from build123d import *

# Parameters (mm, degrees)
F1_DEPTH = 2
F0_W     = 9
F0_H     = 12.07
F0_R     = 1.85
F2_DEPTH = 10


with BuildPart() as f1:
    # F0 (on Top) → F1 (new body)
    with BuildSketch(Plane.XY):
        Polygon((-21.5, -9.07), (-21.5, 0), (-24.5, 0), (-24.5, -12.07), (0, -12.07), (0, -9.07), align=None)
    extrude(amount=F1_DEPTH)

    # F0 (on Top) → F2 (join)
    with BuildSketch(Plane.XY):
        with Locations((-29, -6.035)):
            Rectangle(F0_W, F0_H)
        with Locations((-29.12242, -8.461017)):
            Circle(F0_R, mode=Mode.SUBTRACT)
    extrude(amount=F2_DEPTH)

    # F3: F1 across face


with BuildPart() as f1_1:
    add(f1.part)
    add(f1.part.mirror(Plane(origin=(-28.625, 0, 4.75), x_dir=(-1, 0, 0), z_dir=(0, 1, 0))))

    # F4: F1 across plane


with BuildPart() as f1_2:
    add(f1_1.part)
    add(f1_1.part.mirror(Plane.YZ))


solid = f1_2.part
Part model, mm, in its own coordinate system. A direction names the side the tool comes from. Coordinates: 2 decimals unless noted, no trailing zeros. Loops run counter-clockwise (first coordinate to the right, second up) from the corner with the lowest first, then second, coordinate; pieces in that order, holes last. Notation, with made-up numbers: M -18,13.5 L 35,13.5 A20 cw 35,17.5 Z; hole C 73,22 d8. An arc over 180 degrees is marked long. Use a Markdown table: item, result. Add a question column.
Q1. Cut at D-D (x = -23.5). Write the cut outline in (y, z), and give its area (3 significant figures).
Q2. Cut at A-A (y = 2.75). Write the cut outline in (x, z).
Q3. Cut at B-B (x = 14). Write the cut outline in (y, z), and give its area (3 significant figures).
Q4. Cut at C-C (z = 9.25). Write the cut outline in (x, y).
Q5. Pin check, flat tip, straight feed: P1, Ø12, axis at x = 6, y = 6, coming from the +Z side. Stop position of the tip, or through.
Q6. Mould opens along Y. For faces 1 (the flat face through (0.5, -12.07, 1.6)), 2 (the flat face through (0, 9.07, 1)), 3 (the flat face through (33.5, 0, 5)) say: +Y half, -Y half, draft (parallel to the pull), parting line (faces both ways), or undercut.
Q7. Probe L1, parallel to X at y = 8.25, z = 8.25; L2, parallel to X at y = 7, z = 6.75; L3, parallel to X at y = 0.5, z = 3.75. List the from-to ranges inside material, lowest first.
Q8. Which spindle directions (+Z, -Z, +X, -X, +Y, -Y) get a long thin tool onto all of the face, cutting with end or side? Do faces 4 (the flat face through (-29, 0, 10)), 5 (the flat face through (0, -10, 2)), 6 (the flat face through (21.5, 0, 1)). Say none if no direction does.
Worked out:
| question | item | result |
|---|---|---|
| 1 | outline | M -12.07,0 L 12.07,0 L 12.07,2 L -12.07,2 Z |
| 1 | area | 48.3 mm2 |
| 2 | outline | M -33.5,0 L -21.5,0 L -21.5,2 L -24.5,2 L -24.5,10 L -33.5,10 Z; M 21.5,0 L 33.5,0 L 33.5,10 L 24.5,10 L 24.5,2 L 21.5,2 Z |
| 3 | outline | M -12.07,0 L -9.07,0 L -9.07,2 L -12.07,2 Z; M 9.07,0 L 12.07,0 L 12.07,2 L 9.07,2 Z |
| 3 | area | 12.0 mm2 |
| 4 | outline | M -33.5,-12.07 L -24.5,-12.07 L -24.5,12.07 L -33.5,12.07 Z; M 24.5,-12.07 L 33.5,-12.07 L 33.5,12.07 L 24.5,12.07 Z; hole C -29.12,-8.46 d3.7; hole C -29.12,8.46 d3.7; hole C 29.12,-8.46 d3.7; hole C 29.12,8.46 d3.7 |
| 5 | P1 | stops at z = 2 |
| 6 | face 1 | -Y half |
| 6 | face 2 | undercut |
| 6 | face 3 | draft |
| 7 | L1 | x = -33.5 to -30.96, -27.28 to -24.5, 24.5 to 27.28, 30.96 to 33.5 |
| 7 | L2 | x = -33.5 to -30.26, -27.99 to -24.5, 24.5 to 27.99, 30.26 to 33.5 |
| 7 | L3 | x = -33.5 to -24.5, 24.5 to 33.5 |
| 8 | face 4 | +Z, +X, -X, +Y, -Y |
| 8 | face 5 | +Z, +Y, -Y |
| 8 | face 6 | +Z, -Z |
